Job drawing, mm, ordinate dimensions from the low corner. One solid piece. A direction names the side the tool comes from. Coordinates: 2 decimals unless noted, no trailing zeros. Loops run counter-clockwise (first coordinate to the right, second up) from the corner with the lowest first, then second, coordinate; pieces in that order, holes last. Notation, with made-up numbers: M 12.5,19.25 L 34.5,19.25 A22 cw 34.5,42.25 Z; hole C -26,42.25 d8. An arc over 180 degrees is marked long. Answer as a JSON object with one key per item and string values. Group by question number.
1. Saw through at B-B on y = 54. Write the cut outline in (x, z), then the cut area to 3 significant figures.
2. 3-axis set-ups, long thin cutter, end or side, ignore diameter. For the marked faces 1 and 2: which of +Z, -Z, +X, -X, +Y, -Y reach the whole face in a straight line?
3. Drill centre lines: L1, parallel to Y at x = 7.5, z = 16; L2, parallel to Y at x = 24, z = 43; L3, parallel to X at y = 92.5, z = 39. Where is each one in solid material? Low to high.
4. Saw through at D-D on x = 13. Write the cut outline in (y, z), then the cut area to 3 significant figures.
5. Saw through at A-A on x = 7.5. Write the cut outline in (y, z).
6. Mould opens along X. For the marked faces 3, 4, 5 and 6 say: released by +X, released by -X, zero draft, split by the parting line, or undercut.
7. Saw through at C-C on z = 16.5. Write the cut outline in (x, y).
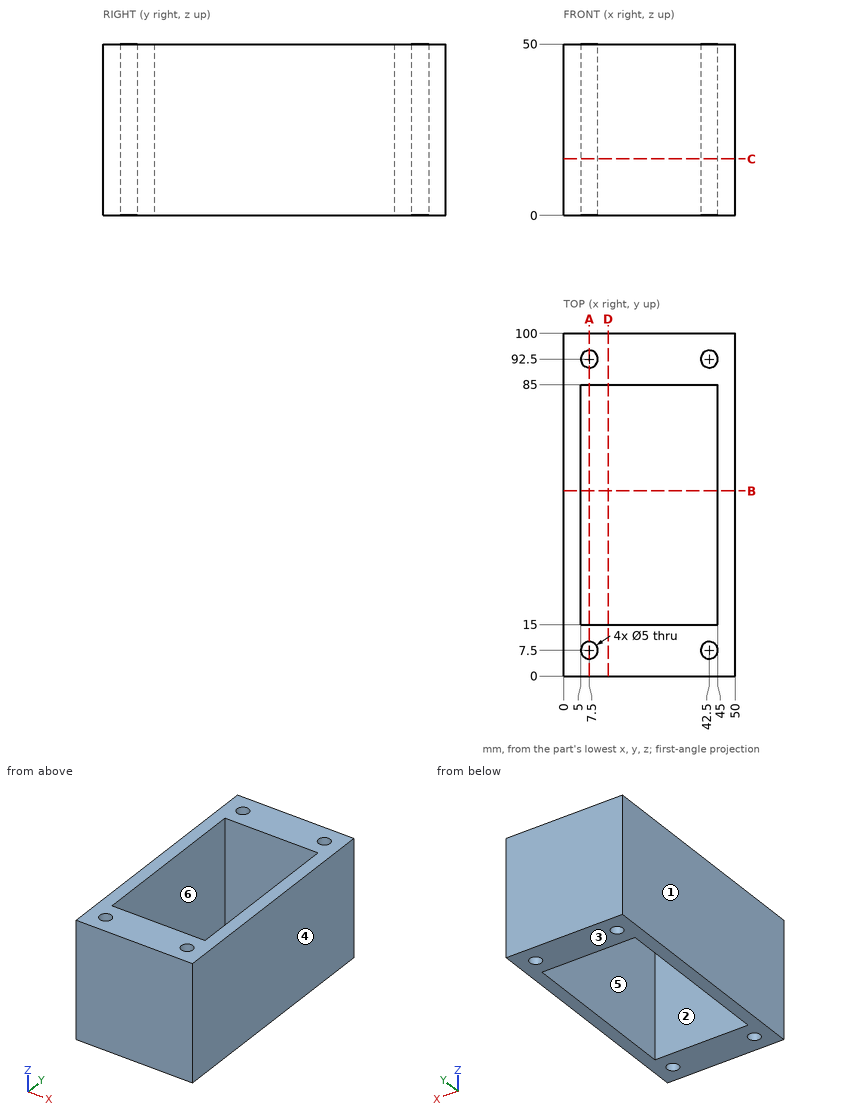
Outcome:
{
 "1": {"outline": "M 0,0 L 5,0 L 5,50 L 0,50 Z; M 45,0 L 50,0 L 50,50 L 45,50 Z", "area": "500 mm²"},
 "2": {"face 1": "+Z, -Z, -X, +Y, -Y", "face 2": "+Z, -Z"},
 "3": {"L1": "y = 0 to 5, 10 to 15, 85 to 90, 95 to 100", "L2": "y = 0 to 15, 85 to 100", "L3": "x = 0 to 5, 10 to 40, 45 to 50"},
 "4": {"outline": "M 0,0 L 15,0 L 15,50 L 0,50 Z; M 85,0 L 100,0 L 100,50 L 85,50 Z", "area": "1,500 mm²"},
 "5": {"outline": "M 0,0 L 5,0 L 5,50 L 0,50 Z; M 10,0 L 15,0 L 15,50 L 10,50 Z; M 85,0 L 90,0 L 90,50 L 85,50 Z; M 95,0 L 100,0 L 100,50 L 95,50 Z"},
 "6": {"face 3": "zero draft", "face 4": "released by +X", "face 5": "undercut", "face 6": "undercut"},
 "7": {"outline": "M 0,0 L 50,0 L 50,100 L 0,100 Z; hole C 7.5,7.5 d5; hole M 5,15 L 45,15 L 45,85 L 5,85 Z; hole C 7.5,92.5 d5; hole C 42.5,7.5 d5; hole C 42.5,92.5 d5"}
}
